Autodesk Inventor part; units mm, degrees
ref_plane "YZ Plane" through (0, 0, 0) normal (1, 0, 0) x (0, 1, 0)
ref_plane "XZ Plane" through (0, 0, 0) normal (0, 1, 0) x (-1, 0, 0)
ref_plane "XY Plane" through (0, 0, 0) normal (0, 0, 1) x (1, 0, 0)
sketch "Sketch1" plane through (0, 0, 0) normal (1, 0, 0) x (0, 1, 0)
  line L0 (0, -5) -> (0, -8)
  line L1 (0, -8) -> (-1.5, -8)
  line L2 (-1.5, -8) -> (-1.5, -6.5)
  line L3 (-1.5, -6.5) -> (-10, -6.5)
  line L4 (-10, -6.5) -> (-10, -5)
  line L5 (-10, -5) -> (0, -5)
  line L6 (0, 5.637) -> (0, -6.8088)
  line L7 (5.7696, 0) -> (-13.4996, 0)
  point P0 (0, 0)
  point P1 (0, -0.5859)
  dimension "d0" = 5
  dimension "d2" = 1.5
  dimension "d3" = 10
  dimension "d4" = 1.5
  dimension "d5" = 8
revolve "Revolution1" add sketch "Sketch1" angle 360 about axis through (0, 5.7696, 0) along (0, -1, 0)
equation "\"d2\" = d4"
properties part number "Flange_Sleeve_Bearing_5448T5" material "Bronze, Cast"
Input: part model. Units: mm. Frame: model coordinates. A direction names the side the tool comes from. Give positions to 0.01 mm unless a question says otherwise; leave off trailing zeros. Write each loop counter-clockwise with the first axis right and the second up, starting at its lowest first coordinate (ties: lowest second). Pieces come first, ordered by that corner, then holes. Notation, with made-up numbers: M 68,-29.5 L 125,-29.5 A5 ccw 125,-25.5 Z; hole C -9,80 d3. An arc over 180 degrees is marked long. Use one line per item in the form item = value.
1. First-contact query: P1, Ø6, axis at x = -6, y = -6.5, coming from the -Z side; P2, Ø1.5, axis at y = -2, z = -5.5, coming from the -X side; P3, Ø1.5, axis at x = 6, y = -8, coming from the -Z side. Flat tips, straight axial feed; report the tip coordinate or a pass-through.
Outcome:
P1 = -5.77
P2 = -6.29
P3 = -3.83
2. Mould query, pull axis Z, two halves, no side actions, for faces 1 (the face through (-7.81, -0.76, 1.73)), 2 (the face through (4.88, -4.93, 1.08)), 3 (the face through (-5, -10, -2)). Classes: released by +Z, released by -Z, zero draft, split by the parting line, or undercut.
Outcome:
face_1 = split by the parting line
face_2 = undercut
face_3 = zero draft
3. Reachability of faces 4 (the face through (-5.2, 0, 0.1)), 5 (the face through (-3.955, -5.81, 5.158)) from +Z, -Z, +X, -X, +Y, -Y: full face, straight path, thin tool, end or side. Return the list, or none.
Outcome:
face_4 = +Z, -Z, +X, -X, +Y
face_5 = -Y
4. Ray query, L1, parallel to X at y = -4.75, z = 0; L2, parallel to Z at x = -1.5, y = -6.75; L3, parallel to Y at x = 0.25, z = -7. Return the intervals inside material, ascending.
Outcome:
L1 = -6.5 to -5, 5 to 6.5
L2 = -6.32 to -4.77, 4.77 to 6.32
L3 = -1.5 to 0
5. Cut plane B-B on z = 0. Return loops of the section in (x, y), and give its area (3 significant figures).
Outcome:
outline = M -8,-1.5 L -6.5,-1.5 L -6.5,-10 L -5,-10 L -5,0 L -8,0 Z; M 5,-10 L 6.5,-10 L 6.5,-1.5 L 8,-1.5 L 8,0 L 5,0 Z
area = 34.5 mm²
6. Cut plane A-A on x = 0. Return loops of the section in (y, z).
Outcome:
outline = M -10,-6.5 L -1.5,-6.5 L -1.5,-8 L 0,-8 L 0,-5 L -10,-5 Z; M -10,5 L 0,5 L 0,8 L -1.5,8 L -1.5,6.5 L -10,6.5 Z
7. Cut plane D-D on z = 5.25. Return loops of the section in (x, y).
Outcome:
outline = M -6.04,-1.5 L -3.83,-1.5 L -3.83,-10 L 3.83,-10 L 3.83,-1.5 L 6.04,-1.5 L 6.04,0 L -6.04,0 Z
8. Cut plane C-C on x = 6.25. Return loops of the section in (y, z).
Outcome:
outline = M -10,-1.79 L -1.5,-1.79 L -1.5,-4.99 L 0,-4.99 L 0,4.99 L -1.5,4.99 L -1.5,1.79 L -10,1.79 Z
